Source: CAD feature listing. Evaluate the final solid. Frame: model axes, mm. Face numbers are marked on the shaded views. A direction names the side the tool comes from. Coordinates: 2 decimals unless noted, no trailing zeros. Order: outer loops, then holes, each group sorted by start corner. A loop starts at its lowest first (then second) coordinate and runs counter-clockwise, first axis right, second up.
Item 1: Section D-D on z = 0.25. Return the cut outline in (x, y).
Item 2: Ray query, line 1 (X direction, y = -4.75, z = 3.25); line 2 (Y direction, x = 14, z = -3.75); line 3 (Y direction, x = 15.5, z = 3.25). Return the intervals inside material, ascending.
Item 3: Mould query, pull axis Y, two halves, no side actions, for the marked faces 1, 2, 3 and 4. Classes: released by +Y, released by -Y, zero draft, split by the parting line, or undercut.
Item 4: Contact query for flat-ended pins moving along their axis: P1, Ø5.5, axis at x = 17, y = -10, coming from the -Z side (3 decimals); P2, Ø1.5, axis at x = 15, y = 10, coming from the -Z side. Output: stop coordinate, or through.
Item 5: Section A-A on z = 2. Return the cut outline in (x, y), then the cut area to 3 significant figures.
Item 6: Reachability of the marked faces 5 and 6 from +Z, -Z, +X, -X, +Y, -Y: full face, straight path, thin tool, end or side. Return the list, or none.
Item 7: Section C-C on x = 12.5. Return the cut outline in (y, z) (3 decimals), then the cut area to 3 significant figures.
Item 8: Section B-B on y = 8.75. Return the cut outline in (x, z) (3 decimals), then the cut area to 3 significant figures.
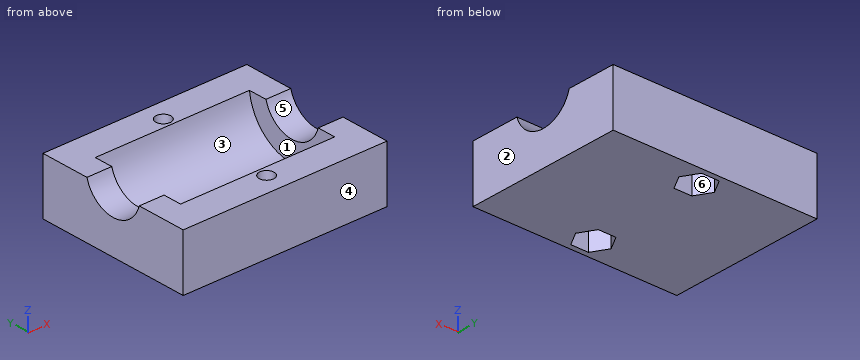
from build123d import *

# Parameters (mm, degrees)
F0_W      = 24.892
F0_H      = 8.89
F1_DEPTH  = 3.937
F3_DEPTH  = 24.4602
F4_W      = 24.892
F4_H      = 8.89
F5_DEPTH  = 3.937
F7_DEPTH  = 32.3352
F8_R      = 1.1811
F9_DEPTH  = 8.891
F11_DEPTH = 3.302


with BuildPart() as f1:
    # F0 (on Right) → F1 (new body)
    with BuildSketch(Plane.YZ):
        Rectangle(F0_W, F0_H)
    extrude(amount=F1_DEPTH)

    # F2 (on face) → F3 (join)
    with BuildSketch(Plane.YZ.offset(3.937)):
        with BuildLine():
            Line((-7.5709045061, 4.445), (-12.446, 4.445))
            Line((-12.446, 4.445), (-12.446, -4.445))
            Line((-12.446, -4.445), (12.446, -4.445))
            Line((12.446, -4.445), (12.446, 4.445))
            Line((12.446, 4.445), (7.5709045061, 4.445))
            ThreePointArc((7.5709045061, 4.445), (0, -2.3114), (-7.5709045061, 4.445))
        make_face()
    extrude(amount=F3_DEPTH)

    # F4 (on face) → F5 (join)
    with BuildSketch(Plane.YZ.offset(28.3972)):
        Rectangle(F4_W, F4_H)
    extrude(amount=F5_DEPTH)

    # F6 (on face) → F7 (cut, through all)
    with BuildSketch(Plane.YZ.offset(32.3342)):
        with BuildLine():
            Line((4.6417414146, 4.445), (-4.6417414146, 4.445))
            ThreePointArc((-4.6417414146, 4.445), (0, 0.9398), (4.6417414146, 4.445))
        make_face()
    extrude(amount=-F7_DEPTH, mode=Mode.SUBTRACT)

    # F8 (on face) → F9 (cut, through all)
    with BuildSketch(Plane.XY.offset(4.445)):
        with Locations((16.1671, -9.1694)):
            Circle(F8_R)
        with Locations((16.1671, 9.1694)):
            Circle(F8_R)
    extrude(amount=-F9_DEPTH, mode=Mode.SUBTRACT)

    # F10 (on face) → F11 (cut)
    with BuildSketch(Plane(origin=(0, 0, -4.445), x_dir=(1, 0, 0), z_dir=(0, 0, -1))):
        Polygon((14.7592891036, -6.731), (13.3514782072, -9.1694), (14.7592891036, -11.6078), (17.5749108964, -11.6078), (18.9827217928, -9.1694), (17.5749108964, -6.731), align=None)
        Polygon((13.3514782072, 9.1694), (14.7592891036, 6.731), (17.5749108964, 6.731), (18.9827217928, 9.1694), (17.5749108964, 11.6078), (14.7592891036, 11.6078), align=None)
    extrude(amount=-F11_DEPTH, mode=Mode.SUBTRACT)


solid = f1.part
Answer list:
1. outline: (0, -12.45) - (32.33, -12.45) - (32.33, 12.45) - (0, 12.45) - close; hole (3.94, -5.7) - (28.4, -5.7) - (28.4, 5.7) - (3.94, 5.7) - close; hole circle Ø2.36 at (16.17, -9.17); hole circle Ø2.36 at (16.17, 9.17)
2. line 1: x = 0 to 3.94, 28.4 to 32.33
2. line 2: y = -12.45 to -10.29, -8.05 to 8.05, 10.29 to 12.45
2. line 3: y = -12.45 to -10.14, -8.19 to -7.34, 7.34 to 8.19, 10.14 to 12.45
3. face 1: undercut
3. face 2: zero draft
3. face 3: undercut
3. face 4: released by -Y
4. P1: stops at z = -4.445
4. P2: stops at z = -1.14
5. outline: (0, -12.45) - (32.33, -12.45) - (32.33, -3.02) - (28.4, -3.02) - (28.4, -6.86) - (3.94, -6.86) - (3.94, -3.02) - (0, -3.02) - close; (0, 3.02) - (3.94, 3.02) - (3.94, 6.86) - (28.4, 6.86) - (28.4, 3.02) - (32.33, 3.02) - (32.33, 12.45) - (0, 12.45) - close; hole circle Ø2.36 at (16.17, -9.17); hole circle Ø2.36 at (16.17, 9.17)
5. area: 413 mm2
6. face 5: +Z, +X, -X
6. face 6: -Z
7. outline: (-12.446, -4.445) - (12.446, -4.445) - (12.446, 4.445) - (7.571, 4.445) arc R7.62 cw to (-7.571, 4.445) - (-12.446, 4.445) - close
7. area: 143 mm2
8. outline: (0, -4.445) - (13.594, -4.445) - (13.594, -1.143) - (15.063, -1.143) - (15.063, 4.445) - (0, 4.445) - close; (17.271, -1.143) - (18.741, -1.143) - (18.741, -4.445) - (32.334, -4.445) - (32.334, 4.445) - (17.271, 4.445) - close
8. area: 258 mm2
